Autodesk Inventor part; units mm, degrees
ref_plane "YZ Plane" through (0, 0, 0) normal (1, 0, 0) x (0, 1, 0)
ref_plane "XZ Plane" through (0, 0, 0) normal (0, 1, 0) x (-1, 0, 0)
ref_plane "XY Plane" through (0, 0, 0) normal (0, 0, 1) x (1, 0, 0)
sketch "Sketch1" plane through (0, 0, 0) normal (0, 0, 1) x (1, 0, 0)
  circle A0 centre (0, 0) radius 13.9
  dimension "d0" = 27.8
extrude "Extrusion1" add sketch "Sketch1" along normal blind 24
fillet "Fillet1" radius 1.5 1 edges at (-13.9, 0, 24)
chamfer "Chamfer1" distance 2 angle 45 1 edges at (-13.9, 0, 0)
sketch "Sketch2" plane through (0, 0, 0) normal (0, 0, -1) x (-1, 0, 0)
  circle A0 centre (0, 0) radius 11.9 construction
  circle A1 centre (0, 0) radius 3.94
  line L0 (0, 0) -> (0, -2.6934)
  line L1 (3.4, -1.9909) -> (3.4, 1.9909)
  line L2 (-3.4, -1.9909) -> (-3.4, 1.9909)
  point P0 (0, -1.3467)
  dimension "d7" = 7.88
  dimension "d8" = 6.8
extrude "Extrusion2" add sketch "Sketch2" along normal blind 14 contours L1 A1 L2
sketch "Sketch3" plane through (0, 0, 24) normal (0, 0, 1) x (1, 0, 0)
  circle A0 centre (0, 0) radius 12.4 construction
  line L0 (0, 0) -> (0, 10.8794)
  line L1 (0, 0) -> (9.5, 0)
  circle A1 centre (9.5, 0) radius 1.5
  circle A2 centre (0, 8) radius 1.5
  circle A3 centre (-9.5, 0) radius 1.5
  circle A4 centre (0, -8) radius 1.5
  dimension "d11" = 8
  dimension "d12" = 9.5
  dimension "d13" = 3
  dimension "d14" = 3
extrude "Extrusion3" cut sketch "Sketch3" against normal blind 4
thread "Thread1"
thread "Thread2"
thread "Thread3"
thread "Thread4"
properties part number "motor"
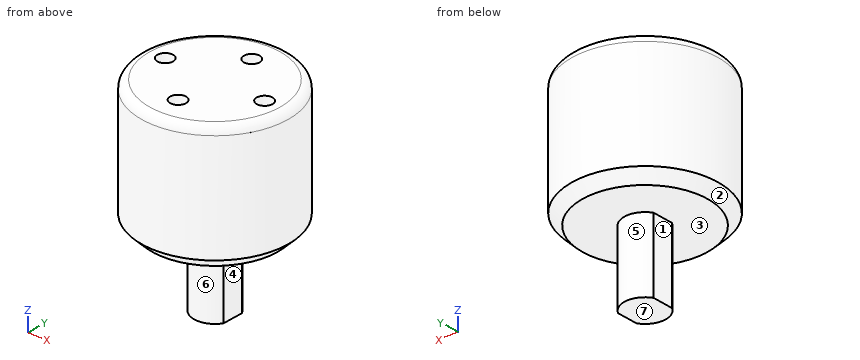
The listing builds one solid part. Answer for the finished solid, in the listing's coordinates (mm). Face numbers are marked on the shaded views. A direction names the side the tool comes from. Round coordinates to 2 decimals unless told otherwise and drop trailing zeros. Loops run counter-clockwise (first coordinate to the right, second up) from the corner with the lowest first, then second, coordinate; pieces in that order, holes last. Notation, with made-up numbers: (7, 31) - (20, 31) arc R23 cw to (20, 42) - close; hole circle Ø11 at (23.25, -34.75). An arc over 180 degrees is marked (long way). Return JSON: item names as keys, results as strings. Group by question number.
1. Each of these flat-tipped pins is pushed along its axis until it touches: P1, Ø4.5, axis at y = 0, z = -6.5, coming from the -X side; P2, Ø1, axis at x = 8.5, y = 0, coming from the -Z side; P3, Ø1, axis at y = -3, z = -1.5, coming from the +X side. Where does it stop, or does it pass through?
2. The part is cut by section A-A on y = 0. Determine the outline of the cut face in (x, z), then the cut area to 3 significant figures.
3. The part is cut by section D-D on z = -0.5. Determine the outline of the cut face in (x, y).
4. The part is cut by section C-C on z = 17.5. Determine the outline of the cut face in (x, y).
5. Which of the six approach directions +Z, -Z, +X, -X, +Y, -Y give full straight-line access (tool end or side, diameter ignored) to the marked faces 5, 6 and 7?
6. The mould has two halves that part along X. Classify the marked faces 1, 2, 3 and 4: pulls with the +X half, pulls with the -X half, needs draft (parallel to the pull), parting line crosses it, or undercut.
7. The part is cut by section B-B on x = 0. Determine the outline of the cut face in (y, z), then the cut area to 3 significant figures.
8. Consider probe 1 along Y at (x, z) = (0, 21.1); probe 2 along Z at (x, y) = (-4.5, 10); probe 3 along Y at (x, z) = (0, -2). Determine where each line is inside the solid, lowest interval first.
Resolved:
{
 "1": {"P1": "stops at x = -3.4", "P2": "stops at z = 0", "P3": "stops at x = 3.05"},
 "2": {"outline": "(-13.9, 2) - (-11.9, 0) - (-3.4, 0) - (-3.4, -14) - (3.4, -14) - (3.4, 0) - (11.9, 0) - (13.9, 2) - (13.9, 22.5) arc R1.5 ccw to (12.4, 24) - (11, 24) - (11, 20) - (8, 20) - (8, 24) - (-8, 24) - (-8, 20) - (-11, 20) - (-11, 24) - (-12.4, 24) arc R1.5 ccw to (-13.9, 22.5) - close", "area": "733 mm²"},
 "3": {"outline": "(-3.4, -1.99) arc R3.94 ccw to (3.4, -1.99) - (3.4, 1.99) arc R3.94 ccw to (-3.4, 1.99) - close"},
 "4": {"outline": "circle Ø27.8 at (0, 0)"},
 "5": {"face 5": "-Z, +Y", "face 6": "-Z, -Y", "face 7": "-Z, +X, -X, +Y, -Y"},
 "6": {"face 1": "pulls with the -X half", "face 2": "parting line crosses it", "face 3": "needs draft", "face 4": "pulls with the +X half"},
 "7": {"outline": "(-13.9, 2) - (-11.9, 0) - (-3.94, 0) - (-3.94, -14) - (3.94, -14) - (3.94, 0) - (11.9, 0) - (13.9, 2) - (13.9, 22.5) arc R1.5 ccw to (12.4, 24) - (9.5, 24) - (9.5, 20) - (6.5, 20) - (6.5, 24) - (-6.5, 24) - (-6.5, 20) - (-9.5, 20) - (-9.5, 24) - (-12.4, 24) arc R1.5 ccw to (-13.9, 22.5) - close", "area": "749 mm²"},
 "8": {"probe 1": "y = -13.9 to -9.5, -6.5 to 6.5, 9.5 to 13.9", "probe 2": "z = 0 to 24", "probe 3": "y = -3.94 to 3.94"}
}
